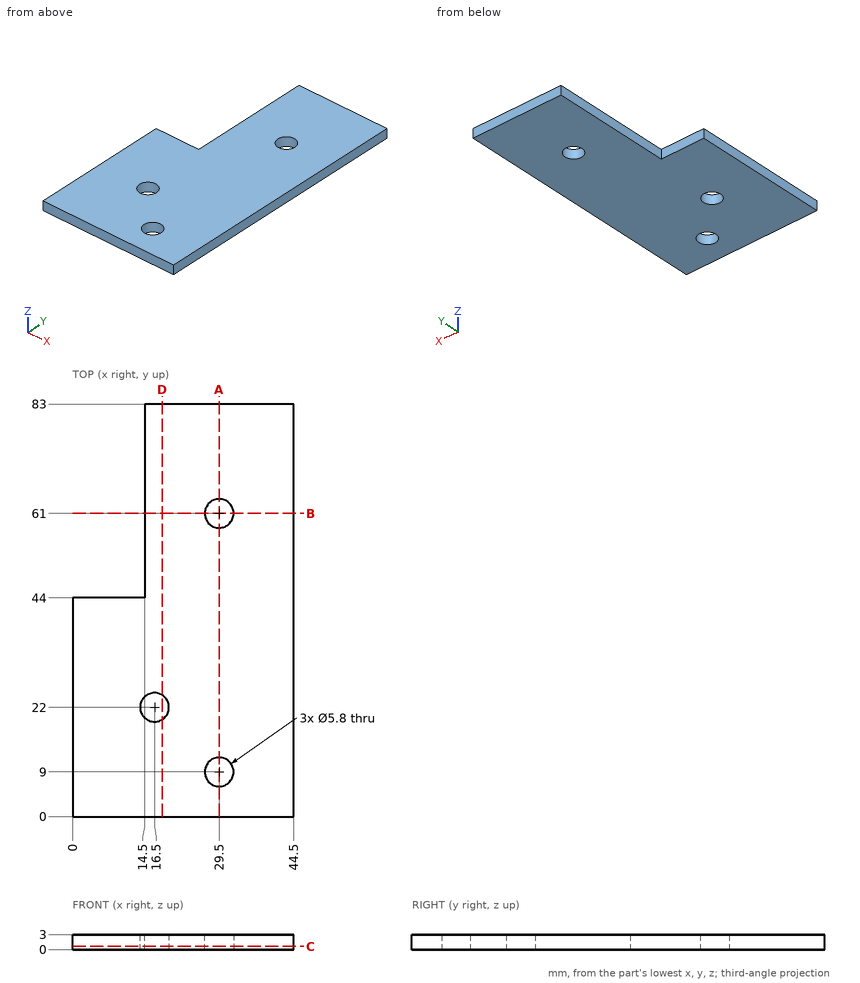
Input: dimensioned drawing with shaded views. Units: mm. Origin: part minimum x, y, z. Give positions to 0.01 mm unless a question says otherwise; leave off trailing zeros. Loops run counter-clockwise (first coordinate to the right, second up) from the corner with the lowest first, then second, coordinate; pieces in that order, holes last. Notation, with made-up numbers: (-21, 58) - (-5, 58) arc R23 cw to (-5, 83) - close; hole circle Ø3 at (77.5, 3). An arc over 180 degrees is marked (long way). Answer as CSV lines item,"result". Start each with the question number.
(1) Section query B-B (y = 61). Output: boundary loops of the cut face in (x, z).
(2) Section query C-C (z = 0.65). Output: boundary loops of the cut face in (x, y), and give its area (3 significant figures).
(3) Pin query (flat end, axial travel): P1, Ø1.5, axis at x = 5.5, z = 1, coming from the +Y side. Return the tip coordinate at first contact, or that it passes through.
(4) Section query D-D (x = 18). Output: boundary loops of the cut face in (y, z), and give its area (3 significant figures).
(5) Section query A-A (x = 29.5). Output: boundary loops of the cut face in (y, z).
(6) Ray query, line 1 along Y through (x, z) = (29.5, 2.05); line 2 along Y through (x, z) = (16.5, 1.75); line 3 along X through (y, z) = (68, 2.4). Return the intervals inside material, ascending. Write a range as [from, to].
Worked answers:
1,outline,"(14.5, 0) - (26.6, 0) - (26.6, 3) - (14.5, 3) - close; (32.4, 0) - (44.5, 0) - (44.5, 3) - (32.4, 3) - close"
2,outline,"(0, 0) - (44.5, 0) - (44.5, 83) - (14.5, 83) - (14.5, 44) - (0, 44) - close; hole circle Ø5.8 at (16.5, 22); hole circle Ø5.8 at (29.5, 9); hole circle Ø5.8 at (29.5, 61)"
2,area,"3,050 mm^2"
3,P1,"stops at y = 44"
4,outline,"(0, 0) - (19.52, 0) - (19.52, 3) - (0, 3) - close; (24.48, 0) - (83, 0) - (83, 3) - (24.48, 3) - close"
4,area,"234 mm^2"
5,outline,"(0, 0) - (6.1, 0) - (6.1, 3) - (0, 3) - close; (11.9, 0) - (58.1, 0) - (58.1, 3) - (11.9, 3) - close; (63.9, 0) - (83, 0) - (83, 3) - (63.9, 3) - close"
6,line 1,"y = [0, 6.1], [11.9, 58.1], [63.9, 83]"
6,line 2,"y = [0, 19.1], [24.9, 83]"
6,line 3,"x = [14.5, 44.5]"
